from build123d import *

# Parameters (mm, degrees)
BOSS_EXTRUDE1_DEPTH = 6
SKETCH3_W           = 20
SKETCH3_H           = 2
CUT_EXTRUDE1_DEPTH  = 6
SKETCH4_R           = 0.75
CUT_EXTRUDE2_DEPTH  = 171.094917366
SKETCH5_R           = 0.75
CUT_EXTRUDE3_DEPTH  = 152.577812455
SKETCH6_R           = 0.75
CUT_EXTRUDE4_DEPTH  = 172.977559331
SKETCH7_R           = 0.75
CUT_EXTRUDE5_DEPTH  = 190.504855499
SKETCH9_R           = 0.75
CUT_EXTRUDE6_DEPTH  = 12
SKETCH10_R          = 1.1
CUT_EXTRUDE7_DEPTH  = 12
SKETCH11_R          = 1.1
CUT_EXTRUDE8_DEPTH  = 12
SKETCH12_R          = 0.75
CUT_EXTRUDE9_DEPTH  = 12
SKETCH15_W          = 20
SKETCH15_H          = 30
BOSS_EXTRUDE4_DEPTH = 4
FILLET4_R           = 4
SKETCH16_W          = 15
SKETCH16_H          = 30
BOSS_EXTRUDE5_DEPTH = 2
FILLET5_R           = 3
FILLET6_DEPTH       = 1.9999999
FILLET6_START       = 148.554137986
FILLET6_2_DEPTH     = 3.0000001
FILLET6_START_2     = 1.99999999
FILLET6_3_DEPTH     = 3.00000001
SKETCH17_R          = 2.1
CUT_EXTRUDE12_DEPTH = 4


with BuildPart() as part:
    # Sketch1 → Boss-Extrude1 (new body)
    with BuildSketch(Plane.XY):
        Polygon((166.554138086, -30.981559499), (166.554138086, -0.981559499), (102.554138086, -0.981559499), (50.592613859, -30.981559499), (-9.407386141, -30.981559499), (-51.833793012, 11.444847372), (-101.833793012, 11.444847372), (-101.833793012, 7.444847372), (-53.490647262, 7.444847372), (-11.06424039, -34.981559499), (51.664410629, -34.981559499), (103.625934856, -4.981559499), (162.554138086, -4.981559499), (162.554138086, -30.981559499), align=None)
    extrude(amount=BOSS_EXTRUDE1_DEPTH)

    # Sketch3 → Cut-Extrude1 (cut)
    with BuildSketch(Plane.XY.offset(6)):
        with Locations((-91.833793012, 8.444847372)):
            Rectangle(SKETCH3_W, SKETCH3_H)
    extrude(amount=-CUT_EXTRUDE1_DEPTH, mode=Mode.SUBTRACT)

    # Sketch4 → Cut-Extrude2 (cut, through all)
    with BuildSketch(Plane(origin=(0, -0.981559499, 0), x_dir=(1, 0, 0), z_dir=(0, 1, 0))):
        with Locations(Location((107.554138086, -3, 0), (0, 0, 180))):
            Circle(SKETCH4_R)
        with Locations(Location((117.554138086, -3, 0), (0, 0, 180))):
            Circle(SKETCH4_R)
        with Locations(Location((127.554138086, -3, 0), (0, 0, 180))):
            Circle(SKETCH4_R)
        with Locations(Location((137.554138086, -3, 0), (0, 0, 180))):
            Circle(SKETCH4_R)
        with Locations(Location((147.554138086, -3, 0), (0, 0, 180))):
            Circle(SKETCH4_R)
        with Locations(Location((157.554138086, -3, 0), (0, 0, 180))):
            Circle(SKETCH4_R)
    extrude(amount=-CUT_EXTRUDE2_DEPTH, mode=Mode.SUBTRACT)

    # Sketch5 → Cut-Extrude3 (cut, through all)
    with BuildSketch(Plane(origin=(26.063562252, -45.143414047, 0), x_dir=(0.8660254037844379, 0.5000000000000013, 0), z_dir=(-0.5000000000000013, 0.8660254037844379, 0))):
        with Locations(Location((33.323709096, -3, 0), (0, 0, 180))):
            Circle(SKETCH5_R)
        with Locations(Location((43.323709096, -3, 0), (0, 0, 180))):
            Circle(SKETCH5_R)
        with Locations(Location((53.323709096, -3, 0), (0, 0, 180))):
            Circle(SKETCH5_R)
        with Locations(Location((63.323709096, -3, 0), (0, 0, 180))):
            Circle(SKETCH5_R)
        with Locations(Location((73.323709096, -3, 0), (0, 0, 180))):
            Circle(SKETCH5_R)
        with Locations(Location((83.323709096, -3, 0), (0, 0, 180))):
            Circle(SKETCH5_R)
    extrude(amount=-CUT_EXTRUDE3_DEPTH, mode=Mode.SUBTRACT)

    # Sketch6 → Cut-Extrude4 (cut, through all)
    with BuildSketch(Plane(origin=(0, -30.981559499, 0), x_dir=(1, 0, 0), z_dir=(0, 1, 0))):
        with Locations(Location((45.592613859, -3, 0), (0, 0, 180))):
            Circle(SKETCH6_R)
        with Locations(Location((35.592613859, -3, 0), (0, 0, 180))):
            Circle(SKETCH6_R)
        with Locations(Location((25.592613859, -3, 0), (0, 0, 180))):
            Circle(SKETCH6_R)
        with Locations(Location((15.592613859, -3, 0), (0, 0, 180))):
            Circle(SKETCH6_R)
        with Locations(Location((5.592613859, -3, 0), (0, 0, 180))):
            Circle(SKETCH6_R)
        with Locations(Location((-4.407386141, -3, 0), (0, 0, 180))):
            Circle(SKETCH6_R)
    extrude(amount=-CUT_EXTRUDE4_DEPTH, mode=Mode.SUBTRACT)

    # Sketch7 → Cut-Extrude5 (cut, through all)
    with BuildSketch(Plane(origin=(-20.19447282, -20.19447282, 0), x_dir=(0, 0, -1), z_dir=(0.7071067811865487, 0.7071067811865464, 0))):
        with Locations(Location((-3, -10.25524428, 0), (0, 0, 90))):
            Circle(SKETCH7_R)
        with Locations(Location((-3, -0.25524428, 0), (0, 0, 90))):
            Circle(SKETCH7_R)
        with Locations(Location((-3, 9.74475572, 0), (0, 0, 90))):
            Circle(SKETCH7_R)
        with Locations(Location((-3, 19.74475572, 0), (0, 0, 90))):
            Circle(SKETCH7_R)
        with Locations(Location((-3, 29.74475572, 0), (0, 0, 90))):
            Circle(SKETCH7_R)
        with Locations(Location((-3, 39.74475572, 0), (0, 0, 90))):
            Circle(SKETCH7_R)
    extrude(amount=-CUT_EXTRUDE5_DEPTH, mode=Mode.SUBTRACT)

    # Sketch9 → Cut-Extrude6 (cut)
    with BuildSketch(Plane(origin=(0, 11.444847372, 0), x_dir=(1, 0, 0), z_dir=(0, 1, 0))):
        with Locations(Location((-56.833793012, -3, 0), (0, 0, 180))):
            Circle(SKETCH9_R)
        with Locations(Location((-66.833793012, -3, 0), (0, 0, 180))):
            Circle(SKETCH9_R)
        with Locations(Location((-76.833793012, -3, 0), (0, 0, 180))):
            Circle(SKETCH9_R)
    extrude(amount=-CUT_EXTRUDE6_DEPTH, mode=Mode.SUBTRACT)

    # Sketch10 → Cut-Extrude7 (cut)
    with BuildSketch(Plane.XZ.offset(-9.444847372)):
        with Locations(Location((-98.833793012, 3, 0), (0, 0, 270))):
            Circle(SKETCH10_R)
    extrude(amount=-CUT_EXTRUDE7_DEPTH, mode=Mode.SUBTRACT)

    # Sketch11 → Cut-Extrude8 (cut)
    with BuildSketch(Plane.XZ.offset(-9.444847372)):
        with Locations(Location((-86.833793012, 3, 0), (0, 0, 270))):
            Circle(SKETCH11_R)
    extrude(amount=-CUT_EXTRUDE8_DEPTH, mode=Mode.SUBTRACT)

    # Sketch12 → Cut-Extrude9 (cut)
    with BuildSketch(Plane.XZ.offset(-9.444847372)):
        with Locations(Location((-92.833793012, 3, 0), (0, 0, 270))):
            Circle(SKETCH12_R)
    extrude(amount=-CUT_EXTRUDE9_DEPTH, mode=Mode.SUBTRACT)

    # Sketch15 → Boss-Extrude4 (add)
    with BuildSketch(Plane(origin=(166.554138086, 0, 0), x_dir=(0, 0, -1), z_dir=(1, 0, 0))):
        with Locations((-16, -15.981559499)):
            Rectangle(SKETCH15_W, SKETCH15_H)
    extrude(amount=-BOSS_EXTRUDE4_DEPTH)

    # Fillet4
    fillet4_edges = [part.edges().sort_by_distance(p)[0] for p in [
        (162.554138086, -2.981559499, 6),
        (162.554138086, -4.981559499, 3),
    ]]
    fillet(fillet4_edges, radius=FILLET4_R)

    # Sketch16 → Boss-Extrude5 (add)
    with BuildSketch(Plane(origin=(0, 0, 0), x_dir=(-1, 0, 0), z_dir=(0, 0, -1))):
        with Locations((-159.054138086, -15.981559499)):
            Rectangle(SKETCH16_W, SKETCH16_H)
    extrude(amount=-BOSS_EXTRUDE5_DEPTH)

    # Fillet5
    # the kernel refuses this fillet: 3 mm, written as the material it adds along each edge
    with BuildSketch(Plane(origin=(158.554138086, -8.981559499, 2), x_dir=(1, 0, 0), z_dir=(0, -1, 0))) as fillet5_piece_1:
        with BuildLine():
            CenterArc((4 - FILLET5_R, FILLET5_R), FILLET5_R, 270, 90)
            Line((4, FILLET5_R), (4, 0))
            Line((4, 0), (4 - FILLET5_R, 0))
        make_face()
    revolve(axis=Axis((158.554138086, -8.981559499, 2), (0, 0, 1)), revolution_arc=90)
    with BuildSketch(Plane(origin=(151.554138086, -4.981559499, 2), x_dir=(0, -1, 0), z_dir=(1, 0, 0))) as fillet5_piece_2_section:
        with BuildLine():
            CenterArc((FILLET5_R, -FILLET5_R), FILLET5_R, 90, 90)
            Line((0, -FILLET5_R), (0, 0))
            Line((0, 0), (FILLET5_R, 0))
        make_face()
    fillet5_piece_2 = extrude(amount=7, mode=Mode.PRIVATE)
    fillet5_piece_2 = fillet5_piece_2 - Plane(origin=(157.554138086, -4.981559499, 3), x_dir=(-1, 0, 0), z_dir=(0, 1, 0)) * Cylinder(0.75, 27, mode=Mode.PRIVATE)
    add(fillet5_piece_2)
    with BuildSketch(Plane(origin=(162.554138086, -8.981559499, 2), x_dir=(0, 0, 1), z_dir=(0, -1, 0))) as fillet5_piece_3:
        with BuildLine():
            CenterArc((FILLET5_R, FILLET5_R), FILLET5_R, 180, 90)
            Line((0, FILLET5_R), (0, 0))
            Line((0, 0), (FILLET5_R, 0))
        make_face()
    extrude(amount=22)

    # Fillet6: read off the stored shape, not the designer's step
    # Fillet6 outline → Fillet6 (add)
    with BuildSketch(Plane.XY):
        with BuildLine():
            ThreePointArc((148.554138086, -4.981559499), (150.67545843, -5.860239155), (151.554138086, -7.981559499))
            Line((151.554138086, -7.981559499), (151.554138086, -4.981559499))
            Line((151.554138086, -4.981559499), (148.554138086, -4.981559499))
        make_face()
    extrude(amount=FILLET6_DEPTH)

    # Fillet6 2 outline → Fillet6 2 (add)
    with BuildSketch(Plane.YZ.offset(FILLET6_START)):
        with BuildLine():
            ThreePointArc((-4.981559499, 5), (-5.860239155, 2.878679656), (-7.981559499, 2))
            Line((-7.981559499, 2), (-4.981559499, 1.9999999))
            Line((-4.981559499, 1.9999999), (-4.981559499, 5))
        make_face()
    extrude(amount=FILLET6_2_DEPTH)

    # Fillet6 3 outline → Fillet6 3 (cut)
    with BuildSketch(Plane.XY.offset(FILLET6_START_2)):
        with BuildLine():
            Line((151.554138085, -9), (151.554138086, -7.981559499))
            ThreePointArc((151.554138086, -7.981559499), (150.67545843, -5.860239155), (148.554138086, -4.981559499))
            Line((148.554138086, -4.981559499), (148.554137986, -9))
            Line((148.554137986, -9), (151.554138085, -9))
        make_face()
    extrude(amount=FILLET6_3_DEPTH, mode=Mode.SUBTRACT)

    # Sketch17 → Cut-Extrude12 (cut)
    with BuildSketch(Plane(origin=(166.554138086, 0, 0), x_dir=(0, 0, -1), z_dir=(1, 0, 0))):
        with Locations(Location((-19, -20.981559499, 0), (0, 0, 90))):
            Circle(SKETCH17_R)
        with Locations(Location((-7, -20.981559499, 0), (0, 0, 90))):
            Circle(SKETCH17_R)
    extrude(amount=-CUT_EXTRUDE12_DEPTH, mode=Mode.SUBTRACT)


solid = part.part
Check sheet for the modelled part. Datum: model origin and axes. Units: mm. A direction names the side the tool comes from. Round coordinates to 2 decimals unless told otherwise and drop trailing zeros. Loops run counter-clockwise (first coordinate to the right, second up) from the corner with the lowest first, then second, coordinate; pieces in that order, holes last. Notation, with made-up numbers: (-36, 74.5) - (-8, 74.5) arc R27 cw to (-8, 102.5) - close; hole circle Ø7 at (-1.75, 86). An arc over 180 degrees is marked (long way). Answer as CSV lines item,"result". Start each with the question number.
Item 1: Depth check by flat-ended pin: P1, Ø2, axis at x = 127.55, z = 3, coming from the +Y side; P2, Ø6.5, axis at x = 154, y = -15, coming from the +Z side; P3, Ø6, axis at y = 1, z = 21.5, coming from the -X side; P4, Ø1.8, axis at x = -98.83, z = 3, coming from the +Y side. Enter the tip coordinate at first touch or a pass-through.
Item 2: Scan lines: line 1 (X direction, y = -9.5, z = 6.75); line 2 (Y direction, x = -23.5, z = 2.5); line 3 (Y direction, x = -22, z = 1.75). Record each from-to range of solid material in increasing order. Write a range as [from, to].
Item 3: Section check A-A (x = 113.5). Record the boundary of the cut face in (y, z).
Item 4: Set-up check for faces 1 (the flat face through (156, -19, 2)), 2 (the flat face through (76.94, -15.77, 2.96)), 3 (the flat face through (-92, 9.445, 4)), 4 (the flat face through (163, -30.982, 10)): record each of +Z, -Z, +X, -X, +Y, -Y from which the full face is reachable in a straight line by a thin tool's end or side.
Item 5: Release check for a two-part mould opening along Y. For faces 5 (the cylindrical face through (164.58, -23.08, 19.09)), 6 (the flat face through (37, -32, 6)), 7 (the cylindrical face through (164.582, -21.255, 9.082)), 8 (the flat face through (125, -4.982, 3)) record: +Y half, -Y half, draft (parallel to the pull), parting line (faces both ways), or undercut.
Report:
1,P1,"stops at y = -0.98"
1,P2,"stops at z = 2"
1,P3,"stops at x = 162.55"
1,P4,"passes through"
2,line 1,"x = [162.55, 166.55]"
2,line 2,"y = [-22.55, -16.89]"
2,line 3,"y = [-24.05, -18.39]"
3,outline,"(-4.98, 0) - (-0.98, 0) - (-0.98, 6) - (-4.98, 6) - close"
4,face 1,"+Z, -Y"
4,face 2,"+Z, -Z, +Y"
4,face 3,"+Z, -Z, -X, -Y"
4,face 4,"+Z, -Z, +X, -Y"
5,face 5,"undercut"
5,face 6,"draft"
5,face 7,"undercut"
5,face 8,"-Y half"
